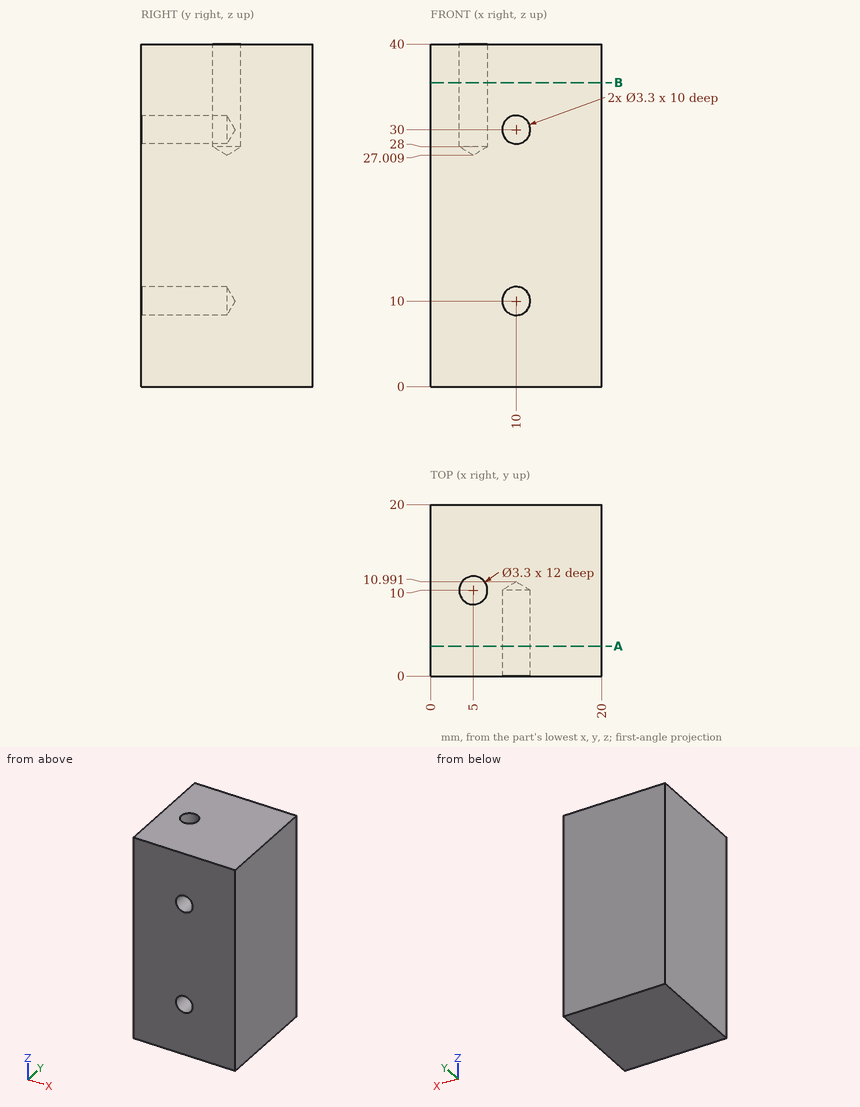
Design review of the part shown in the three views and the two pictorial views. Dimensions are in mm from the part's minimum x, y and z. Round coordinates to 2 decimals unless told otherwise and drop trailing zeros. Loops run counter-clockwise (first coordinate to the right, second up) from the corner with the lowest first, then second, coordinate; pieces in that order, holes last. Notation, with made-up numbers: (52, 62) - (98, 62) arc R17 cw to (98, 74) - close; hole circle Ø7 at (19, 62). An arc over 180 degrees is marked (long way). Use one line per item in the form item = value.
1) We need section B-B on z = 35.5. Write out the cut boundary in (x, y).
Solutions:
outline = (0, 0) - (20, 0) - (20, 20) - (0, 20) - close; hole circle Ø3.3 at (5, 10)
2) Wall thickness on probe 1 along Z at (x, y) = (10, 3); probe 2 along X at (y, z) = (1, 11); probe 3 along X at (y, z) = (11, 35.5): over which ranges is each line inside the solid? List them lowest first.
Solutions:
probe_1 = 0 to 8.35, 11.65 to 28.35, 31.65 to 40
probe_2 = 0 to 8.69, 11.31 to 20
probe_3 = 0 to 3.69, 6.31 to 20
3) We need section A-A on y = 3.5. Write out the cut boundary in (x, z).
Solutions:
outline = (0, 0) - (20, 0) - (20, 40) - (0, 40) - close; hole circle Ø3.3 at (10, 10); hole circle Ø3.3 at (10, 30)
